```python
from build123d import *

# Parameters (mm, degrees)
SKETCH2_R          = 39
SKETCH2_R_2        = 10.5
CUT_EXTRUDE1_DEPTH = 1.5
FILLET1_R          = 0.75
CUT_EXTRUDE2_DEPTH = 1.5
FILLET2_R          = 3.5


with BuildPart() as part:
    # Sketch1 → Revolve1 (revolve)
    with BuildSketch(Plane.XY, mode=Mode.PRIVATE) as revolve1_sk:
        Polygon((-3.5, 6), (-3.5, 0), (-45, 0), (-43.5, 1.5), (-45, 3), (-7.5, 3), (-6, 4.5), (-7.5, 6), align=None)
    revolve(revolve1_sk.sketch.rotate(Axis((0, 0, 0), (0, 1, 0)), 270), axis=Axis((0, 0, 0), (0, 1, 0)))

    # Sketch2 → Cut-Extrude1 (cut)
    with BuildSketch(Plane(origin=(0, 3, 0), x_dir=(1, 0, 0), z_dir=(0, 1, 0))):
        with Locations(Location((0, 0, 0), (0, 0, 270))):
            Circle(SKETCH2_R)
        with Locations(Location((0, 0, 0), (0, 0, 270))):
            Circle(SKETCH2_R_2, mode=Mode.SUBTRACT)
    extrude(amount=-CUT_EXTRUDE1_DEPTH, mode=Mode.SUBTRACT)

    # Fillet1
    fillet1_edges = [part.edges().sort_by_distance(p)[0] for p in [
        (0, 1.5, -10.5),
        (0, 1.5, -39),
    ]]
    fillet(fillet1_edges, radius=FILLET1_R)
    fillet1_2_edges = [part.edges().sort_by_distance(p)[0] for p in [
        (0, 3, -39),
        (0, 3, -10.5),
    ]]
    fillet(fillet1_2_edges, radius=FILLET1_R - 0.0001)  # a hair under: the kernel refuses the full size

    # Sketch3 → Cut-Extrude2 (cut)
    with BuildSketch(Plane(origin=(0, 1.5, 0), x_dir=(1, 0, 0), z_dir=(0, 1, 0))):
        with BuildLine():
            Line((35.398622855, -5), (12.808688457, -5))
            ThreePointArc((12.808688457, -5), (9.722718241, -9.722718241), (5, -12.808688457))
            Line((5, -12.808688457), (5, -35.398622855))
            ThreePointArc((5, -35.398622855), (25.279067427, -25.279067427), (35.398622855, -5))
        make_face()
        with BuildLine():
            Line((-5, -35.398622855), (-5, -12.808688457))
            ThreePointArc((-5, -12.808688457), (-9.722718241, -9.722718241), (-12.808688457, -5))
            Line((-12.808688457, -5), (-35.398622855, -5))
            ThreePointArc((-35.398622855, -5), (-25.279067427, -25.279067427), (-5, -35.398622855))
        make_face()
        with BuildLine():
            Line((-35.398622855, 5), (-12.808688457, 5))
            ThreePointArc((-12.808688457, 5), (-9.722718241, 9.722718241), (-5, 12.808688457))
            Line((-5, 12.808688457), (-5, 35.398622855))
            ThreePointArc((-5, 35.398622855), (-25.279067427, 25.279067427), (-35.398622855, 5))
        make_face()
        with BuildLine():
            Line((5, 35.398622855), (5, 12.808688457))
            ThreePointArc((5, 12.808688457), (9.722718241, 9.722718241), (12.808688457, 5))
            Line((12.808688457, 5), (35.398622855, 5))
            ThreePointArc((35.398622855, 5), (25.279067427, 25.279067427), (5, 35.398622855))
        make_face()
    extrude(amount=-CUT_EXTRUDE2_DEPTH, mode=Mode.SUBTRACT)

    # Fillet2
    fillet2_edges = [part.edges().sort_by_distance(p)[0] for p in [
        (5, 0.75, -35.398622855),
        (35.398622855, 0.75, -5),
        (12.808688457, 0.75, -5),
        (5, 0.75, -12.808688457),
        (-5, 0.75, -12.808688457),
        (-12.808688457, 0.75, -5),
        (-35.398622855, 0.75, -5),
        (-5, 0.75, -35.398622855),
        (-12.808688457, 0.75, 5),
        (-5, 0.75, 12.808688457),
        (-5, 0.75, 35.398622855),
        (-35.398622855, 0.75, 5),
        (35.398622855, 0.75, 5),
        (5, 0.75, 35.398622855),
        (5, 0.75, 12.808688457),
        (12.808688457, 0.75, 5),
    ]]
    fillet(fillet2_edges, radius=FILLET2_R)


solid = part.part
```
Check sheet for the modelled part. Datum: model origin and axes. Units: mm. A direction names the side the tool comes from. Round coordinates to 2 decimals unless told otherwise and drop trailing zeros. Write item = value, one per line. Start each with the question number.
1. Gauge pin test, flat ends, axial feed: pin 1 (3 mm diameter, centred on x = 26.5, y = 4, fed in from +Z); pin 2 (4 mm diameter, centred on x = 28, z = -2, fed in from -Y); pin 3 (1.5 mm diameter, centred on y = 3.5, z = 30, fed in from +X); pin 4 (0.8 mm diameter, centred on x = -26, y = 1, fed in from -Z). Record the tip position at first contact, or that the pin passes through.
2. Release check for a two-part mould opening along Z. For faces 4 (the cylindrical face through (3.417, 2.958, 0.759)), 5 (the cylindrical face through (33.864, 0.74, 6.341)), 6 (the flat face through (9, 0, -1)) record: pulls with the +Z half, pulls with the -Z half, needs draft (parallel to the pull), parting line crosses it, or undercut.
3. Scan lines: line 1 (X direction, y = 0.3, z = 13.5); line 2 (X direction, y = 2.3, z = 0); line 3 (Y direction, x = 26, z = -34). Record each from-to range of solid material in increasing order. Write a range as [from, to].
4. Section check C-C, the plane x = -28. State how many separate pieces and enclosed holes the cut face has, then the cut area to 3 significant figures.
5. Tool access check on faces 1 (the flat face through (-11, 1.5, 3)), 2 (the cylindrical face through (6.341, 0.74, 33.864)), 3 (the flat face through (-1.8, 6, -3.2)). Record the directions out of +Z, -Z, +X, -X, +Y, -Y that give a thin tool (end or side, any length) a straight path to the whole face; none if there is none.
Results found:
q1.pin_1 = 37.16
q1.pin_2 = 0
q1.pin_3 = 34.03
q1.pin_4 = -36.07
q2.face_4 = undercut
q2.face_5 = undercut
q2.face_6 = needs draft
q3.line_1 = [-42.61, -33.1], [-5.34, 5.34], [33.1, 42.61]
q3.line_2 = [-44.3, -39], [-10.5, -3.5], [3.5, 10.5], [39, 44.3]
q3.line_3 = [0, 3]
q4.separate_pieces = 3
q4.enclosed_holes = 0
q4.area = 72.5 mm^2
q5.face_1 = +Y
q5.face_2 = +Y, -Y
q5.face_3 = +Z, -Z, +X, -X, +Y
